from build123d import *

# Parameters (mm, degrees)
SKETCH1_R          = 866.025405
EXTRUDE1_DEPTH     = 20
SKETCH2_R          = 75
CUT_EXTRUDE1_DEPTH = 10


# Read off the part's stored shape, not the designer's step: 连接重组1
with BuildPart() as part:
    # Sketch1 → Extrude1 (new body)
    with BuildSketch(Plane(origin=(0, 0, 0), x_dir=(1, 0, 0), z_dir=(0, 1, 0))):
        with Locations(Location((0, 0, 0), (0, 0, 270))):
            Circle(SKETCH1_R)
    extrude(amount=-EXTRUDE1_DEPTH)

    # Sketch2 → Cut-Extrude1 (cut)
    with BuildSketch(Plane(origin=(0, 0, 0), x_dir=(1, 0, 0), z_dir=(0, 1, 0))):
        with Locations(Location((0, 606.2177835, 0), (0, 0, 270))):
            Circle(SKETCH2_R)
        with Locations(Location((290.671285018, 531.987034708, 0), (0, 0, 270))):
            Circle(SKETCH2_R)
        with Locations(Location((525.000000737, -303.10889175, 0), (0, 0, 270))):
            Circle(SKETCH2_R)
        with Locations(Location((315.378644033, -517.72223433, 0), (0, 0, 270))):
            Circle(SKETCH2_R)
        with Locations(Location((-525.000000737, -303.10889175, 0), (0, 0, 270))):
            Circle(SKETCH2_R)
        with Locations(Location((-606.04992905, -14.264800378, 0), (0, 0, 270))):
            Circle(SKETCH2_R)
    extrude(amount=-CUT_EXTRUDE1_DEPTH, mode=Mode.SUBTRACT)

    # 连接重组1 outline → 连接重组1 (revolve)
    with BuildSketch(Plane.XY.offset(-606.2177835)):
        with BuildLine():
            Line((75, 75), (34.641016131, 75.000000035))
            ThreePointArc((34.641016131, 75.000000035), (34.641016161, 35.000000018), (0, 15))
            Line((0, 15), (0, -10))
            Line((0, -10), (75, -10))
            Line((75, -10), (75, 75))
        make_face()
    revolve(axis=Axis((0, 0, -606.2177835), (0, 1, 0)))

    # Other 1 2 outline → Other 1 2 (revolve)
    with BuildSketch(Plane(origin=(290.671285018, 0, -531.987034708), x_dir=(1, 0, 0), z_dir=(0, 0, 1))):
        with BuildLine():
            Line((75, 75), (34.641016131, 75.000000035))
            ThreePointArc((34.641016131, 75.000000035), (34.641016161, 35.000000018), (0, 15))
            Line((0, 15), (0, -10))
            Line((0, -10), (75, -10))
            Line((75, -10), (75, 75))
        make_face()
    revolve(axis=Axis((290.671285018, 0, -531.987034708), (0, 1, 0)))

    # Other 1 3 outline → Other 1 3 (revolve)
    with BuildSketch(Plane(origin=(315.378644033, 0, 517.72223433), x_dir=(1, 0, 0), z_dir=(0, 0, 1))):
        with BuildLine():
            Line((75, 75), (34.641016131, 75.000000035))
            ThreePointArc((34.641016131, 75.000000035), (34.641016161, 35.000000018), (0, 15))
            Line((0, 15), (0, -10))
            Line((0, -10), (75, -10))
            Line((75, -10), (75, 75))
        make_face()
    revolve(axis=Axis((315.378644033, 0, 517.72223433), (0, 1, 0)))

    # Other 1 4 outline → Other 1 4 (revolve)
    with BuildSketch(Plane(origin=(-525.000000737, 0, 303.10889175), x_dir=(1, 0, 0), z_dir=(0, 0, 1))):
        with BuildLine():
            Line((75, 75), (34.641016131, 75.000000035))
            ThreePointArc((34.641016131, 75.000000035), (34.641016161, 35.000000018), (0, 15))
            Line((0, 15), (0, -10))
            Line((0, -10), (75, -10))
            Line((75, -10), (75, 75))
        make_face()
    revolve(axis=Axis((-525.000000737, 0, 303.10889175), (0, 1, 0)))

    # Other 1 5 outline → Other 1 5 (revolve)
    with BuildSketch(Plane(origin=(-606.04992905, 0, 14.264800378), x_dir=(1, 0, 0), z_dir=(0, 0, 1))):
        with BuildLine():
            Line((75, 75), (34.641016131, 75.000000035))
            ThreePointArc((34.641016131, 75.000000035), (34.641016161, 35.000000018), (0, 15))
            Line((0, 15), (0, -10))
            Line((0, -10), (75, -10))
            Line((75, -10), (75, 75))
        make_face()
    revolve(axis=Axis((-606.04992905, 0, 14.264800378), (0, 1, 0)))

    # Other 1 6 outline → Other 1 6 (revolve)
    with BuildSketch(Plane(origin=(525.000000737, 0, 303.10889175), x_dir=(1, 0, 0), z_dir=(0, 0, 1))):
        with BuildLine():
            Line((75, 75), (34.641016131, 75.000000035))
            ThreePointArc((34.641016131, 75.000000035), (34.641016161, 35.000000018), (0, 15))
            Line((0, 15), (0, -10))
            Line((0, -10), (75, -10))
            Line((75, -10), (75, 75))
        make_face()
    revolve(axis=Axis((525.000000737, 0, 303.10889175), (0, 1, 0)))


solid = part.part
Build history of the part. All positions in model axes, mm. A direction names the side the tool comes from. Give positions to 0.01 mm unless a question says otherwise; leave off trailing zeros. Order: outer loops, then holes, each group sorted by start corner. A loop starts at its lowest first (then second) coordinate and runs counter-clockwise, first axis right, second up. Notation, with made-up numbers: M -22.5,89.25 L 1.5,89.25 A4 ccw 1.5,94.25 Z; hole C -16,53.25 d10. An arc over 180 degrees is marked long. Use one line per item in the form item = value.
1) Saw through at C-C (x = 704). Give the cut face in (y, z), plus the area to 3 significant figures.
Calculated:
outline = M -20,-504.36 L 0,-504.36 L 0,504.36 L -20,504.36 Z
area = 20,200 mm2
2) Two-plate mould, pull along Z, no slides. Class faces 1 (the face through (280.91, 38.02, -606.35)), 2 (the face through (-453.463, 38.025, 280.581)), 3 (the face through (12, -20, -12)), 4 (the face through (-331.69, -9.86, 799.99)): released by +Z, released by -Z, zero draft, split by the parting line, or undercut.
Calculated:
face_1 = undercut
face_2 = undercut
face_3 = zero draft
face_4 = split by the parting line
3) Probe probe 1 along Y at (x, z) = (792, -275.5); probe 2 along Z at (x, y) = (-579, 41); probe 3 along X at (y, z) = (38.5, 510). List the from-to ranges inside material, lowest first.
Calculated:
probe_1 = -20 to 0
probe_2 = -55.69 to -11.66, 40.19 to 84.22, 251.06 to 355.16
probe_3 = 240.78 to 279.77, 350.99 to 389.98
4) Saw through at B-B (z = 734). Give the cut face in (x, y), plus the area to 3 significant figures.
Calculated:
outline = M -459.61,-20 L 459.61,-20 L 459.61,0 L -459.61,0 Z
area = 18,400 mm2
5) Drop flat-ended pins along their axis: pin 1 (12 mm diameter, centred on y = 60, z = 482.5, fed in from +X); pin 2 (3 mm diameter, centred on y = 42, z = 372, fed in from +X); pin 3 (1 mm diameter, centred on x = 410.5, z = -25, fed in from +Y). Give the stop position or say it passes through.
Calculated:
pin_1 = 384.45
pin_2 = 557.92
pin_3 = 0
6) Saw through at A-A (y = 42). State how many separate pieces and enclosed holes the cut face has, plus the area to 3 significant figures.
Calculated:
separate_pieces = 6
enclosed_holes = 6
area = 79,100 mm2
7) Tool access for faces 5 (the face through (-574, 75, 30)), 6 (the face through (12, 0, -12)): list every direction of +Z, -Z, +X, -X, +Y, -Y with a clear straight run to the whole face (end or side of a thin tool).
Calculated:
face_5 = +Z, -Z, +X, -X, +Y
face_6 = +Y
